from build123d import *

# Parameters (mm, degrees)
SKETCH1_R           = 3.3
SKETCH1_R_2         = 27.5
SKETCH1_R_3         = 52.3875
SKETCH1_R_4         = 2
BOSS_EXTRUDE1_DEPTH = 11.43


with BuildPart() as part:
    # Sketch1 → Boss-Extrude1 (new body)
    with BuildSketch(Plane(origin=(0, 0, 0), x_dir=(1, 0, 0), z_dir=(0, 1, 0))):
        with BuildLine():
            Line((-455.030211447, -196.569220819), (-601.269315712, -129.028875319))
            ThreePointArc((-601.269315712, -129.028875319), (-611.168375764, -123.292603215), (-619.842929594, -115.832822829))
            ThreePointArc((-619.842929594, -115.832822829), (-625.62049557, -111.271620388), (-632.402453753, -108.409823836))
            Line((-632.402453753, -108.409823836), (-661.891152149, -106.785342117))
            ThreePointArc((-661.891152149, -106.785342117), (-670.303863855, -100.570549133), (-667.940742704, -90.381681261))
            Line((-667.940742704, -90.381681261), (-654.343117313, -77.414452829))
            ThreePointArc((-654.343117313, -77.414452829), (-650.072978561, -70.012815509), (-650.805846426, -61.499224923))
            Line((-650.805846426, -61.499224923), (-673.057822329, -18.34288652))
            ThreePointArc((-673.057822329, -18.34288652), (-672.544957076, -8.73610108), (-663.918846707, -4.476573271))
            Line((-663.918846707, -4.476573271), (-570.934950003, -11.063752399))
            ThreePointArc((-570.934950003, -11.063752399), (-561.986230526, -12.359631359), (-553.321698813, -14.945124108))
            ThreePointArc((-553.321698813, -14.945124108), (-545.349986654, -17.107158275), (-537.109590399, -17.671477372))
            Line((-537.109590399, -17.671477372), (-451.561292182, -15.180486069))
            ThreePointArc((-451.561292182, -15.180486069), (-445.839616936, -16.885847624), (-442.257047488, -21.661936169))
            Line((-442.257047488, -21.661936169), (-399.995822112, -147.172985144))
            ThreePointArc((-399.995822112, -147.172985144), (-411.258692171, -189.980718354), (-455.030211447, -196.569220819))
        make_face()
        with Locations(Location((-661.367230642, -97.274762153, 0), (0, 0, 270))):
            Circle(SKETCH1_R, mode=Mode.SUBTRACT)
        with Locations(Location((-664.591931322, -13.977761728, 0), (0, 0, 270))):
            Circle(SKETCH1_R, mode=Mode.SUBTRACT)
        with Locations(Location((-451.284061184, -24.701450725, 0), (0, 0, 270))):
            Circle(SKETCH1_R, mode=Mode.SUBTRACT)
        with Locations(Location((-438.15, -160.02, 0), (0, 0, 270))):
            Circle(SKETCH1_R_2, mode=Mode.SUBTRACT)
        with Locations(Location((-575.31, -72.821477372, 0), (0, 0, 270))):
            Circle(SKETCH1_R_3, mode=Mode.SUBTRACT)
        with Locations(Location((-632.402453753, -70.257452317, 0), (0, 0, 270))):
            Circle(SKETCH1_R_4, mode=Mode.SUBTRACT)
        with BuildLine():
            ThreePointArc((-575.31, -17.671477372), (-573.31, -15.671477372), (-575.31, -13.671477372))
            ThreePointArc((-575.31, -13.671477372), (-577.31, -15.671477372), (-575.31, -17.671477372))
        make_face(mode=Mode.SUBTRACT)
        with BuildLine():
            ThreePointArc((-518.217546247, -72.257452317), (-516.217546247, -70.257452317), (-518.217546247, -68.257452317))
            ThreePointArc((-518.217546247, -68.257452317), (-520.217546247, -70.257452317), (-518.217546247, -72.257452317))
        make_face(mode=Mode.SUBTRACT)
        with BuildLine():
            ThreePointArc((-575.31, -131.971477372), (-573.31, -129.971477372), (-575.31, -127.971477372))
            ThreePointArc((-575.31, -127.971477372), (-577.31, -129.971477372), (-575.31, -131.971477372))
        make_face(mode=Mode.SUBTRACT)
    extrude(amount=BOSS_EXTRUDE1_DEPTH)


solid = part.part
Input: part model. Units: mm. Frame: model coordinates. A direction names the side the tool comes from. Coordinates: 2 decimals unless noted, no trailing zeros. Loops run counter-clockwise (first coordinate to the right, second up) from the corner with the lowest first, then second, coordinate; pieces in that order, holes last. Notation, with made-up numbers: (-0.5, 60.5) -> (34.5, 60.5) arc R25 ccw to (34.5, 95.5) -> close; hole circle Ø3 at (19.5, -28). An arc over 180 degrees is marked (long way). Write item = value, one per line. Start each with the question number.
Item 1: Cut plane A-A, the plane z = 142. Return loops of the section in (x, y).
Item 2: Cut plane C-C, the plane y = 5.75. Count the separate pieces of the cut face and the enclosed holes in it, plus the area to 3 significant figures.
Item 3: First-contact query: P1, Ø6, axis at x = -538, y = 3, coming from the +Z side; P2, Ø6, axis at x = -664.59, z = 13.98, coming from the +Y side; P3, Ø10.5, axis at x = -661.37, z = 97.27, coming from the -Y side; P4, Ø3, axis at x = -452, y = 3.5, coming from the -Z side. Flat tips, straight axial feed; report the tip coordinate or a pass-through.
Item 4: Material intervals for line 1 (X direction, y = 9, z = 145); line 2 (X direction, y = 1, z = 82); line 3 (X direction, y = 8, z = 72), sorted ascending.
Item 5: Reachability of faces 5 (the face through (-625.532, 5.635, 111.324)), 6 (the face through (-661.24, 5.63, 83.99)), 7 (the face through (-545.46, 5.63, 17.09)) from +Z, -Z, +X, -X, +Y, -Y: full face, straight path, thin tool, end or side. Return the list, or none.
Item 6: Mould query, pull axis Z, two halves, no side actions, for faces 1 (the face through (-445.91, 5.635, 16.838)), 2 (the face through (-503, 0, 101)), 3 (the face through (-523.37, 5.63, 66)), 4 (the face through (-454.212, 5.635, 26.224)). Classes: pulls with the +Z half, pulls with the -Z half, needs draft (parallel to the pull), parting line crosses it, or undercut.
Item 7: Cut plane B-B, the plane x = -528.5. Return loops of the section in (y, z).
Ans:
q1.outline = (-573.18, 0) -> (-458.92, 0) -> (-458.92, 11.43) -> (-573.18, 11.43) -> close; (-417.38, 0) -> (-401.74, 0) -> (-401.74, 11.43) -> (-417.38, 11.43) -> close
q2.separate_pieces = 1
q2.enclosed_holes = 9
q2.area = 24,000 mm²
q3.P1 = 159.64
q3.P2 = through
q3.P3 = 0
q3.P4 = 15.18
q4.line_1 = -566.69 to -461.19, -415.11 to -400.73
q4.line_2 = -659.15 to -626.89, -523.73 to -421.94
q4.line_3 = -650.67 to -633.38, -631.42 to -627.69, -522.93 to -519.2, -517.24 to -425.31
q5.face_5 = +Z, -X, +Y, -Y
q5.face_6 = -X, +Y, -Y
q5.face_7 = -Z, +Y, -Y
q6.face_1 = pulls with the -Z half
q6.face_2 = needs draft
q6.face_3 = undercut
q6.face_4 = undercut
q7.outline = (0, 17.42) -> (11.43, 17.42) -> (11.43, 49.3) -> (0, 49.3) -> close; (0, 96.34) -> (11.43, 96.34) -> (11.43, 162.64) -> (0, 162.64) -> close
